Geometry: final body of the model. Coordinates: model frame, mm. A direction names the side the tool comes from. Give positions to 0.01 mm unless a question says otherwise; leave off trailing zeros. Order: outer loops, then holes, each group sorted by start corner. A loop starts at its lowest first (then second) coordinate and runs counter-clockwise, first axis right, second up. Notation, with made-up numbers: (-10.5, -34) -> (39.5, -34) arc R13 ccw to (39.5, -23) -> close; hole circle Ø10 at (3.5, -28.75). An arc over 180 degrees is marked (long way). Write item = value, one per line.
```python
from build123d import *

# Parameters (mm, degrees)
SKETCH1_W                          = 150
SKETCH1_H                          = 65
BODY_DEPTH                         = 4
EDGE_FILLETS_R                     = 5
SKETCH5_W                          = 98.5
SKETCH5_H                          = 40.5
LCD2004_SCREEN_CUTOUT_DEPTH        = 82.836727696
LCD2004_MOUNTING_HOLES_START       = 2
LCD2004_MOUNTING_HOLES_OUTLINE_R   = 3.25
LCD2004_MOUNTING_HOLES_DEPTH       = 2
LCD2004_MOUNTING_HOLES_2_OUTLINE_R = 1.6
LCD2004_MOUNTING_HOLES_2_DEPTH     = 2
SKETCH8_W                          = 50
SKETCH8_H                          = 9.75
LCD2004_SOLDERING_CUTOUT_DEPTH     = 2


# Read off the part's stored shape, not the designer's step: mounting_holes, lcd2004_mounting_holes
with BuildPart() as part:
    # Sketch1 → body (new body)
    with BuildSketch(Plane(origin=(0, 0, 0), x_dir=(1, 0, 0), z_dir=(0, 1, 0))):
        Rectangle(SKETCH1_W, SKETCH1_H)
    extrude(amount=BODY_DEPTH)

    # mounting_holes outline → mounting_holes (revolve, cut)
    with BuildSketch(Plane(origin=(70, 0, 27.5), x_dir=(1, 0, 0), z_dir=(0, 0, 1))):
        Polygon((0, 0), (1.7, 0), (1.7, 2), (3.25, 2), (3.25, 3.975), (3.275, 4), (0, 4), align=None)
    revolve(axis=Axis((70, 0, 27.5), (0, 1, 0)), mode=Mode.SUBTRACT)

    # mounting_holes 2 outline → mounting_holes 2 (revolve, cut)
    with BuildSketch(Plane(origin=(-70, 0, -27.5), x_dir=(1, 0, 0), z_dir=(0, 0, 1))):
        Polygon((0, 4), (0, 0), (1.7, 0), (1.7, 2), (3.25, 2), (3.25, 3.975), (3.275, 4), align=None)
    revolve(axis=Axis((-70, 0, -27.5), (0, 1, 0)), mode=Mode.SUBTRACT)

    # mounting_holes 3 outline → mounting_holes 3 (revolve, cut)
    with BuildSketch(Plane(origin=(70, 0, -27.5), x_dir=(1, 0, 0), z_dir=(0, 0, 1))):
        Polygon((0, 4), (0, 0), (1.7, 0), (1.7, 2), (3.25, 2), (3.25, 3.975), (3.275, 4), align=None)
    revolve(axis=Axis((70, 0, -27.5), (0, 1, 0)), mode=Mode.SUBTRACT)

    # mounting_holes 4 outline → mounting_holes 4 (revolve, cut)
    with BuildSketch(Plane(origin=(-70, 0, 27.5), x_dir=(1, 0, 0), z_dir=(0, 0, 1))):
        Polygon((0, 4), (0, 0), (1.7, 0), (1.7, 2), (3.25, 2), (3.25, 3.975), (3.275, 4), align=None)
    revolve(axis=Axis((-70, 0, 27.5), (0, 1, 0)), mode=Mode.SUBTRACT)

    # edge_fillets
    edge_fillets_edges = [part.edges().sort_by_distance(p)[0] for p in [
        (75, 2, 32.5),
        (-75, 2, 32.5),
        (-75, 2, -32.5),
        (75, 2, -32.5),
    ]]
    fillet(edge_fillets_edges, radius=EDGE_FILLETS_R)

    # Sketch5 → lcd2004_screen_cutout (cut, through all)
    with BuildSketch(Plane(origin=(0, 4, 0), x_dir=(1, 0, 0), z_dir=(0, 1, 0))):
        with Locations((11, 0)):
            Rectangle(SKETCH5_W, SKETCH5_H)
    extrude(amount=-LCD2004_SCREEN_CUTOUT_DEPTH, mode=Mode.SUBTRACT)

    # lcd2004_mounting_holes outline → lcd2004_mounting_holes (cut)
    with BuildSketch(Plane(origin=(0, 0, 0), x_dir=(1, 0, 0), z_dir=(0, 1, 0)).offset(LCD2004_MOUNTING_HOLES_START)):
        with Locations((57.5, 27.5)):
            Circle(LCD2004_MOUNTING_HOLES_OUTLINE_R)
        with Locations((-35.5, -27.5)):
            Circle(LCD2004_MOUNTING_HOLES_OUTLINE_R)
        with Locations((57.5, -27.5)):
            Circle(LCD2004_MOUNTING_HOLES_OUTLINE_R)
        with Locations((-35.5, 27.5)):
            Circle(LCD2004_MOUNTING_HOLES_OUTLINE_R)
    extrude(amount=LCD2004_MOUNTING_HOLES_DEPTH, mode=Mode.SUBTRACT)

    # lcd2004_mounting_holes 2 outline → lcd2004_mounting_holes 2 (cut)
    with BuildSketch(Plane(origin=(0, 0, 0), x_dir=(1, 0, 0), z_dir=(0, 1, 0))):
        with Locations((57.5, 27.5)):
            Circle(LCD2004_MOUNTING_HOLES_2_OUTLINE_R)
        with Locations((-35.5, -27.5)):
            Circle(LCD2004_MOUNTING_HOLES_2_OUTLINE_R)
        with Locations((57.5, -27.5)):
            Circle(LCD2004_MOUNTING_HOLES_2_OUTLINE_R)
        with Locations((-35.5, 27.5)):
            Circle(LCD2004_MOUNTING_HOLES_2_OUTLINE_R)
    extrude(amount=LCD2004_MOUNTING_HOLES_2_DEPTH, mode=Mode.SUBTRACT)

    # Sketch8 → lcd2004_soldering_cutout (cut)
    with BuildSketch(Plane.XZ):
        with Locations((29, 25.125)):
            Rectangle(SKETCH8_W, SKETCH8_H)
    extrude(amount=-LCD2004_SOLDERING_CUTOUT_DEPTH, mode=Mode.SUBTRACT)


solid = part.part
```
1) Section query D-D (x = 57.5). Output: boundary loops of the cut face in (y, z), plus the area to 3 significant figures.
Check sheet entries:
outline = (0, -32.5) -> (4, -32.5) -> (4, -30.75) -> (2, -30.75) -> (2, -29.1) -> (0, -29.1) -> close; (0, -25.9) -> (2, -25.9) -> (2, -24.25) -> (4, -24.25) -> (4, -20.25) -> (0, -20.25) -> close; (0, 20.25) -> (4, 20.25) -> (4, 24.25) -> (2, 24.25) -> (2, 25.9) -> (0, 25.9) -> close; (0, 29.1) -> (2, 29.1) -> (2, 30.75) -> (4, 30.75) -> (4, 32.5) -> (0, 32.5) -> close
area = 59.2 mm²
2) Section query B-B (y = 0.8). Count the separate pieces of the cut face and the enclosed holes in it, plus the area to 3 significant figures.
Check sheet entries:
separate_pieces = 1
enclosed_holes = 9
area = 5,180 mm²
3) Section query C-C (x = -29.5). Output: boundary loops of the cut face in (y, z).
Check sheet entries:
outline = (0, -32.5) -> (4, -32.5) -> (4, -20.25) -> (0, -20.25) -> close; (0, 20.25) -> (4, 20.25) -> (4, 32.5) -> (0, 32.5) -> close
4) First-contact query: P1, Ø3, axis at x = -34, z = -27, coming from the +Y side; P2, Ø10, axis at x = 9, z = 17, coming from the -Y side. Flat tips, straight axial feed; report the tip coordinate or a pass-through.
Check sheet entries:
P1 = 2
P2 = 2
5) Reachability of faces 1 (the face through (73.5, 2.03, 31.07)), 2 (the face through (10.3, 2.5, 20.25)), 3 (the face through (67.421, 3.001, -25.522)) from +Z, -Z, +X, -X, +Y, -Y: full face, straight path, thin tool, end or side. Return the list, or none.
Check sheet entries:
face_1 = +Z, +X, +Y, -Y
face_2 = +Y, -Y
face_3 = +Y
6) Mould query, pull axis X, two halves, no side actions, for faces 4 (the face through (-1, 2, -32.5)), 5 (the face through (75, 2, 0)), 6 (the face through (59, 2, 29)). Classes: +X half, -X half, draft (parallel to the pull), parting line (faces both ways), or undercut.
Check sheet entries:
face_4 = draft
face_5 = +X half
face_6 = undercut
7) Line query: line 1 (Z direction, x = 57.5, y = 2.85); line 2 (X direction, y = 1.65, z = 27.5); line 3 (X direction, y = 3.45, z = -27.5). Output: solid intervals per line, ascending. Write a range as from..to.
Check sheet entries:
line_1 = -32.5..-30.75, -24.25..-20.25, 20.25..24.25, 30.75..32.5
line_2 = -75..-71.7, -68.3..-37.1, -33.9..4, 54..55.9, 59.1..68.3, 71.7..75
line_3 = -75..-73.25, -66.75..-38.75, -32.25..54.25, 60.75..66.75, 73.25..75
8) Section query A-A (z = -12). Output: boundary loops of the cut face in (x, y), plus the area to 3 significant figures.
Check sheet entries:
outline = (-75, 0) -> (-38.25, 0) -> (-38.25, 4) -> (-75, 4) -> close; (60.25, 0) -> (75, 0) -> (75, 4) -> (60.25, 4) -> close
area = 206 mm²
